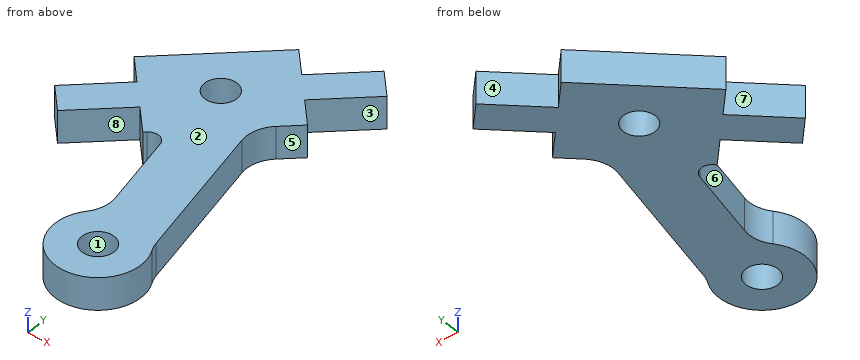
```python
from build123d import *

# Parameters (mm, degrees)
ESQUISSE15_R        = 1.5
BOSS_EXTRU_15_DEPTH = 3


with BuildPart() as part:
    # Esquisse15 → Boss.-Extru.15 (new body)
    with BuildSketch(Plane.XY):
        with BuildLine():
            Line((159.079156624, -48.365258544), (150.563075986, -56.819628453))
            Line((150.563075986, -56.819628453), (152.676668463, -58.948648613))
            Line((152.676668463, -58.948648613), (148.418628144, -63.175833567))
            Line((148.418628144, -63.175833567), (150.532220621, -65.304853727))
            Line((150.532220621, -65.304853727), (154.790260941, -61.077668772))
            Line((154.790260941, -61.077668772), (156.903853418, -63.206688932))
            Line((156.903853418, -63.206688932), (157.114961916, -62.997110206))
            ThreePointArc((157.114961916, -62.997110206), (158.090398383, -62.744177685), (158.790743402, -63.468724451))
            Line((158.790743402, -63.468724451), (160.499830137, -70.44157839))
            ThreePointArc((160.499830137, -70.44157839), (160.521490891, -71.774910136), (159.963165383, -72.985907807))
            ThreePointArc((159.963165383, -72.985907807), (162.875303574, -79.417825737), (166.589129616, -73.413026553))
            ThreePointArc((166.589129616, -73.413026553), (166.3998932, -73.026858147), (166.267814939, -72.617600535))
            Line((166.267814939, -72.617600535), (162.983107766, -59.220583964))
            ThreePointArc((162.983107766, -59.220583964), (163.008961454, -57.693583939), (163.783215914, -56.377176889))
            Line((163.783215914, -56.377176889), (165.419934056, -54.752319023))
            Line((165.419934056, -54.752319023), (163.306341579, -52.623298863))
            Line((163.306341579, -52.623298863), (167.564381898, -48.396113909))
            Line((167.564381898, -48.396113909), (165.450789421, -46.267093749))
            Line((165.450789421, -46.267093749), (161.192749102, -50.494278704))
            Line((161.192749102, -50.494278704), (159.079156624, -48.365258544))
        make_face()
        with Locations((157.991505021, -55.785973738)):
            Circle(ESQUISSE15_R, mode=Mode.SUBTRACT)
        with Locations((163.132615018, -75.426110464)):
            Circle(ESQUISSE15_R, mode=Mode.SUBTRACT)
    extrude(amount=BOSS_EXTRU_15_DEPTH)


solid = part.part
```
Check sheet for the modelled part. Datum: model origin and axes. Units: mm. Face numbers are marked on the shaded views. A direction names the side the tool comes from. Coordinates: 2 decimals unless noted, no trailing zeros. Order: outer loops, then holes, each group sorted by start corner. A loop starts at its lowest first (then second) coordinate and runs counter-clockwise, first axis right, second up. Notation, with made-up numbers: M -36.5,-8 L -22.5,-8 A32 ccw -22.5,29 Z; hole C 39,-30 d2. An arc over 180 degrees is marked long. Write each question's results on one line, items separated by ' | '. Start each with the question number.
1. Go/stop test with flat-tipped pins: P1, Ø1, axis at x = 155.5, z = 0.5, coming from the +Y side; P2, Ø1.5, axis at x = 152.5, z = 1.5, coming from the +Y side; P3, Ø1.5, axis at x = 154, z = 2, coming from the +Y side. Record where each tip stops, or that it passes through.
2. Material ranges on probe 1 along X at (y, z) = (-63, 0.55); probe 2 along X at (y, z) = (-49.5, 1.55); probe 3 along X at (y, z) = (-56.5, 2.3), recorded low to high.
3. Cross-section at B-B on x = 151.5. Record the cut outline in (y, z), and give its area (3 significant figures).
4. Cross-section at C-C on z = 1.95. Record the cut outline in (x, y).
5. Cross-section at A-A on y = -76. Record the cut outline in (x, z).
6. Access from +Z, -Z, +X, -X, +Y, -Y to the whole of each face (thin tool, end or side, straight path). Record for the marked faces 5, 6, 7 and 8.
7. Mould release check, pull along Y, two halves, no side actions. Record for the marked faces 1, 2, 3 and 4: +Y half, -Y half, draft (parallel to the pull), parting line (faces both ways), or undercut.
8. Cross-section at D-D on y = -68.5. Record the cut outline in (x, z), and give its area (3 significant figures).
Checks:
1) P1: stops at y = -51.42 | P2: stops at y = -54.15 | P3: stops at y = -52.66
2) probe 1: x = 148.6 to 152.85, 156.7 to 157.11, 158.53 to 163.91 | probe 2: x = 157.94 to 160.21, 162.19 to 166.45 | probe 3: x = 150.89 to 156.67, 159.31 to 163.67
3) outline: M -64.34,0 L -60.12,0 L -60.12,3 L -64.34,3 Z; M -57.76,0 L -55.89,0 L -55.89,3 L -57.76,3 Z | area: 18.3 mm²
4) outline: M 148.42,-63.18 L 150.53,-65.3 L 154.79,-61.08 L 156.9,-63.21 L 157.11,-63 A1 cw 158.79,-63.47 L 160.5,-70.44 A3 cw 159.96,-72.99 A4 ccw long 166.59,-73.41 A3 cw 166.27,-72.62 L 162.98,-59.22 A3 cw 163.78,-56.38 L 165.42,-54.75 L 163.31,-52.62 L 167.56,-48.4 L 165.45,-46.27 L 161.19,-50.49 L 159.08,-48.37 L 150.56,-56.82 L 152.68,-58.95 Z; hole C 157.99,-55.79 d3; hole C 163.13,-75.43 d3
5) outline: M 159.17,0 L 161.75,0 L 161.75,3 L 159.17,3 Z; M 164.52,0 L 167.09,0 L 167.09,3 L 164.52,3 Z
6) face 5: +Z, -Z, +X | face 6: +Z, -Z | face 7: +Z, -Z, -X | face 8: +Z, -Z, -Y
7) face 1: undercut | face 2: draft | face 3: undercut | face 4: +Y half
8) outline: M 160.02,0 L 165.26,0 L 165.26,3 L 160.02,3 Z | area: 15.7 mm²
